Read the model definition and answer for the solid it produces. Units are mm, in the model's axes. Face numbers are marked on the shaded views. A direction names the side the tool comes from. Round coordinates to 2 decimals unless told otherwise and drop trailing zeros. Write each loop counter-clockwise with the first axis right and the second up, starting at its lowest first coordinate (ties: lowest second). Pieces come first, ordered by that corner, then holes. Notation, with made-up numbers: (85, 34) - (109, 34) arc R6 cw to (109, 40) - close; hole circle Ø2 at (-10, 40). An arc over 180 degrees is marked (long way). One line per item, written item: value. Start each with the question number.
(1) Find the intervals of material crossed by L1, parallel to X at y = -0.2, z = -3.25; L2, parallel to Z at x = -0.2, y = 1.7; L3, parallel to Y at x = -1.25, z = -6, in increasing order.
(2) For the marked faces 1, 2 and 3, determine the directions among +Z, -Z, +X, -X, +Y, -Y from which every point of the face is accessible in a straight line to the end or side of a thin tool.
(3) Flat-ended cylindrical pins translate along their axes: pin 1 Ø2 at (x, z) = (-1, -4) entering from +Y; pin 2 Ø0.5 at (y, z) = (0, -5.5) entering from -X; pin 3 Ø0.6 at (x, z) = (-1.5, -5) entering from -Y. Find the tip coordinate at first contact, or state that the pin passes through.
(4) A cutting plane is placed at D-D, the plane x = 1.2. Determine the outline of the cut face in (y, z), plus the area to 3 significant figures.
(5) A cutting plane is placed at B-B, the plane x = 0. Determine the outline of the cut face in (y, z).
(6) A cutting plane is placed at C-C, the plane y = -0.9. Determine the outline of the cut face in (x, z), plus the area to 3 significant figures.
(7) A cutting plane is placed at A-A, the plane z = -3.75. Determine the outline of the cut face in (x, y).
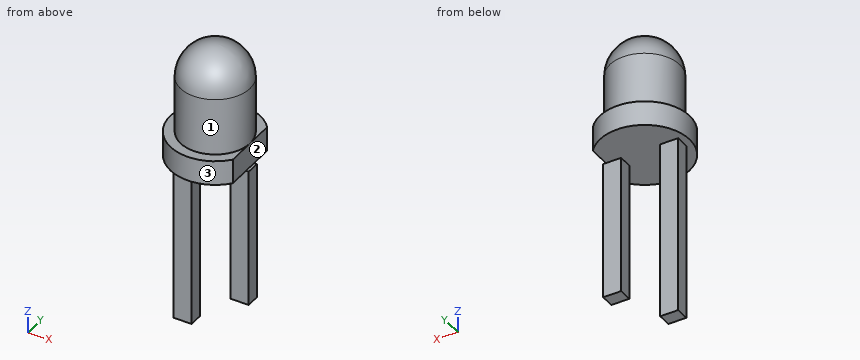
Autodesk Inventor part; units mm, degrees
ref_plane "Arbeitsebene1" through (1.55, 0, 2.375) normal (1, 0, 0) x (0, 1, 0)
ref_plane "XZ Plane" through (0, 0, 0) normal (0, 1, 0) x (-1, 0, 0)
ref_plane "XY Plane" through (0, 0, 0) normal (0, 0, 1) x (1, 0, 0)
sketch "Skizze2" plane through (0, 0, 0) normal (0, 1, 0) x (-1, 0, 0)
  line L0 (0, 0) -> (0, 5.2)
  arc A0 (0, 5.2) -> (-1.55, 3.65) centre (0, 3.65) ccw
  line L1 (-1.55, 3.65) -> (-1.55, 1.1)
  line L2 (-1.55, 1.1) -> (-2, 1.1)
  line L3 (-2, 1.1) -> (-2, 0)
  line L4 (-2, 0) -> (0, 0)
  dimension "d0" = 5.2
  dimension "d1" = 3.1
  dimension "d2" = 4.1
  dimension "d3" = 4
revolve "Umdrehung1" add sketch "Skizze2" angle 360 about axis through (0, 0, 0) along (0, 0, 1)
ref_plane "Arbeitsebene1" through (1.55, 0, 2.375) normal (1, 0, 0) x (0, 1, 0)
sketch "Skizze3" plane through (1.55, 0, 2.375) normal (1, 0, 0) x (0, 1, 0)
  line L0 (2, -2.375) -> (-2, -2.375)
  line L1 (2, -1.275) -> (-2, -1.275)
  line L2 (2, -1.275) -> (-2, -1.275)
  line L3 (-2, -1.275) -> (2, -1.275)
  line L4 (2, -1.275) -> (2, -2.375)
  line L5 (2, -2.375) -> (-2, -2.375)
  line L6 (-2, -2.375) -> (-2, -1.275)
  point P0 (0, -2.375)
extrude "Extrusion1" cut sketch "Skizze3" along normal through all
sketch "Skizze4" plane through (0, 0, 0) normal (0, 1, 0) x (-1, 0, 0)
  line L0 (-1.55, 0) -> (-1.55, 0)
  line L1 (2, 0) -> (-1.55, 0)
  line L2 (0.87, 0) -> (1.67, 0)
  line L3 (1.67, 0) -> (1.67, -8)
  line L4 (1.67, -8) -> (0.87, -8)
  line L5 (0.87, -8) -> (0.87, 0)
  line L6 (-1.67, 0) -> (-0.87, 0)
  line L7 (-0.87, 0) -> (-0.87, -6.2)
  line L8 (-0.87, -6.2) -> (-1.67, -6.2)
  line L9 (-1.67, -6.2) -> (-1.67, 0)
  line L10 (0, -7.8775) -> (0, 7.3796)
  line L11 (1.27, -8) -> (1.27, 0) construction
  line L12 (-1.27, 0) -> (-1.27, -6.2) construction
  point P0 (0, 0)
  dimension "d7" = 0.8
  dimension "d8" = 0.8
  dimension "d9" = 2.54
  dimension "d10" = 1.8
  dimension "d11" = 8
extrude "Extrusion2" add sketch "Skizze4" along normal mid plane 0.6
sketch "Skizze5" plane through (0, 0, 0) normal (1, 0, 0) x (0, 1, 0)
  line L0 (0, 12.04) -> (0, -35.84)
  line L1 (0, 2.4) -> (0, 52.4)
  line L2 (0, 2.4) -> (18.1985, 52.4)
  line L3 (18.1985, 52.4) -> (0, 52.4)
  arc A0 (1.55, 3.65) -> (-1.55, 3.65) centre (0, 3.65) ccw
  line L4 (-3.0679, 5.2) -> (3.702, 5.2) construction
  point P0 (0, 0)
  dimension "d14" = 50
  dimension "d15" = 2.8
  dimension "d16" = 20
revolve "Umdrehung2" [suppressed]
properties part number "LED 3mm" material "PC/ABS-Kunststoff"
Here are the results:
1. L1: -1.67 to -0.87, 0.87 to 1.67
1. L2: 0 to 1.1
1. L3: -0.3 to 0.3
2. face 1: +Z
2. face 2: +Z, +X, +Y, -Y
2. face 3: +Z, -Z
3. pin 1: y = 0.3
3. pin 2: x = -1.67
3. pin 3: y = -0.3
4. outline: (-1.6, 0) - (-0.3, 0) - (-0.3, -6.2) - (0.3, -6.2) - (0.3, 0) - (1.6, 0) - (1.6, 1.1) - (0.98, 1.1) - (0.98, 3.65) arc R0.98 ccw to (-0.98, 3.65) - (-0.98, 1.1) - (-1.6, 1.1) - close
4. area: 13.8 mm²
5. outline: (-2, 0) - (2, 0) - (2, 1.1) - (1.55, 1.1) - (1.55, 3.65) arc R1.55 ccw to (-1.55, 3.65) - (-1.55, 1.1) - (-2, 1.1) - close
6. outline: (-1.79, 0) - (1.55, 0) - (1.55, 1.1) - (1.26, 1.1) - (1.26, 3.65) arc R1.26 ccw to (-1.26, 3.65) - (-1.26, 1.1) - (-1.79, 1.1) - close
6. area: 12.6 mm²
7. outline: (-1.67, -0.3) - (-0.87, -0.3) - (-0.87, 0.3) - (-1.67, 0.3) - close; (0.87, -0.3) - (1.67, -0.3) - (1.67, 0.3) - (0.87, 0.3) - close
